Verification items for this drawing (mm, ordinates from the low corner). A direction names the side the tool comes from. Coordinates: 2 decimals unless noted, no trailing zeros. Write each loop counter-clockwise with the first axis right and the second up, starting at its lowest first coordinate (ties: lowest second). Pieces come first, ordered by that corner, then holes. Notation, with made-up numbers: (48, 65) -> (61, 65) arc R16 ccw to (61, 89) -> close; hole circle Ø7 at (72.25, -16.75). An arc over 180 degrees is marked (long way). Use CSV: the item, a comma, the result in double quotes.
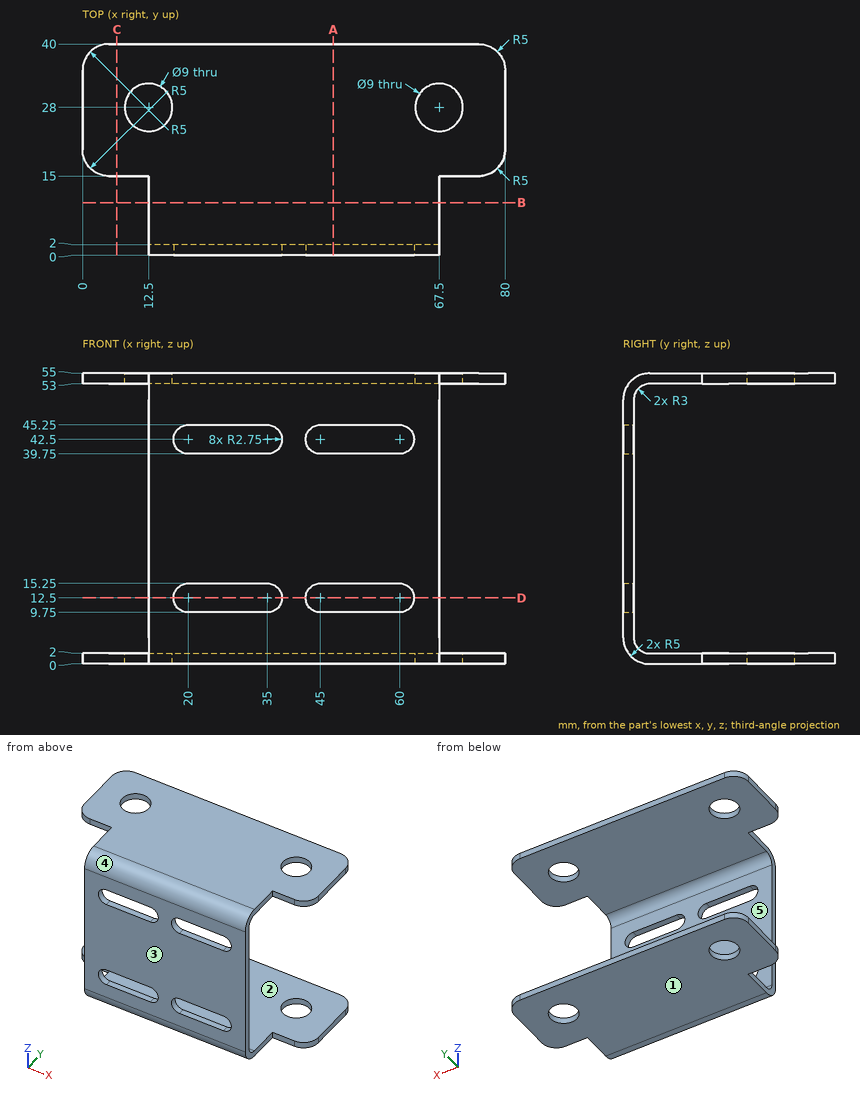
1) Cross-section at A-A (x = 47.5). Record the boundary of the cut face in (y, z), plus the area to 3 significant figures.
Return value:
outline,"(0, 5) arc R5 ccw to (5, 0) -> (40, 0) -> (40, 2) -> (5, 2) arc R3 cw to (2, 5) -> (2, 9.75) -> (0, 9.75) -> close; (0, 15.25) -> (2, 15.25) -> (2, 39.75) -> (0, 39.75) -> close; (0, 45.25) -> (2, 45.25) -> (2, 50) arc R3 cw to (5, 53) -> (40, 53) -> (40, 55) -> (5, 55) arc R5 ccw to (0, 50) -> close"
area,"233 mm2"
2) Cross-section at D-D (z = 12.5). Record the boundary of the cut face in (x, y).
Return value:
outline,"(12.5, 0) -> (17.25, 0) -> (17.25, 2) -> (12.5, 2) -> close; (37.75, 0) -> (42.25, 0) -> (42.25, 2) -> (37.75, 2) -> close; (62.75, 0) -> (67.5, 0) -> (67.5, 2) -> (62.75, 2) -> close"
3) Set-up check for the marked faces 1 and 2: record each of +Z, -Z, +X, -X, +Y, -Y from which the full face is reachable in a straight line by a thin tool's end or side.
Return value:
face 1,"-Z, +X, -X, +Y, -Y"
face 2,"+X, -X, +Y"
4) Cross-section at C-C (x = 6.5). Record the boundary of the cut face in (y, z).
Return value:
outline,"(15, 0) -> (40, 0) -> (40, 2) -> (15, 2) -> close; (15, 53) -> (40, 53) -> (40, 55) -> (15, 55) -> close"
5) Mould release check, pull along Z, two halves, no side actions. Record for the marked faces 3, 4 and 5: released by +Z, released by -Z, zero draft, split by the parting line, or undercut.
Return value:
face 3,"zero draft"
face 4,"released by +Z"
face 5,"undercut"
6) Scan lines: L1, parallel to Z at x = 35, y = 28; L2, parallel to Z at x = 59.5, y = 3; L3, parallel to Y at x = 17.5, z = 44.5. Record each from-to range of solid material in increasing order.
Return value:
L1,"0 to 2, 53 to 55"
L2,"0.42 to 2.76, 52.24 to 54.58"
L3,"0 to 2"
7) Gauge pin test, flat ends, axial feed: pin 1 (0.6 mm diameter, centred on x = 70.5, z = 1.5, fed in from -Y); pin 2 (4 mm diameter, centred on x = 27, z = 29.5, fed in from +Y); pin 3 (2 mm diameter, centred on x = 25, y = 1.5, fed in from -Z); pin 4 (8 mm diameter, centred on x = 12.5, y = 28, fed in from +Z). Record the tip position at first contact, or that the pin passes through.
Return value:
pin 1,"y = 15"
pin 2,"y = 2"
pin 3,"z = 0.67"
pin 4,"through"
8) Cross-section at B-B (y = 10). Record the boundary of the cut face in (x, z).
Return value:
outline,"(12.5, 0) -> (67.5, 0) -> (67.5, 2) -> (12.5, 2) -> close; (12.5, 53) -> (67.5, 53) -> (67.5, 55) -> (12.5, 55) -> close"
